```python
from build123d import *

# Parameters (mm, degrees)
BOSS_EXTRUDE2_DEPTH = 20
BOSS_EXTRUDE3_DEPTH = 2
BOSS_EXTRUDE4_START = 20
BOSS_EXTRUDE4_DEPTH = 2
CUT_EXTRUDE1_DEPTH  = 5
CUT_EXTRUDE2_DEPTH  = 5


with BuildPart() as part:
    # Sketch1 → Boss-Extrude2 (new body)
    with BuildSketch(Plane(origin=(0, 0, 0), x_dir=(0, 0, -1), z_dir=(1, 0, 0))):
        Polygon((0, 28), (0, 0), (28, 0), (28, 4), (4, 4), (4, 28), align=None)
    extrude(amount=BOSS_EXTRUDE2_DEPTH)

    # Sketch1_4 → Boss-Extrude3 (add)
    with BuildSketch(Plane(origin=(0, 0, 0), x_dir=(0, 0, -1), z_dir=(1, 0, 0))):
        Polygon((9.768810499, 28), (4, 28), (4, 4), (28, 4), (28, 9.768810499), (23.299944734, 9.768810499), (9.768810499, 23.299944734), align=None)
    extrude(amount=BOSS_EXTRUDE3_DEPTH)

    # Sketch1_5 → Boss-Extrude4 (add)
    with BuildSketch(Plane(origin=(0, 0, 0), x_dir=(0, 0, -1), z_dir=(1, 0, 0)).offset(BOSS_EXTRUDE4_START)):
        Polygon((9.768810499, 28), (4, 28), (4, 4), (28, 4), (28, 9.768810499), (23.299944734, 9.768810499), (9.768810499, 23.299944734), align=None)
    extrude(amount=-BOSS_EXTRUDE4_DEPTH)

    # Sketch2 → Cut-Extrude1 (cut, through all)
    with BuildSketch(Plane(origin=(0, 4, 0), x_dir=(1, 0, 0), z_dir=(0, 1, 0))):
        with BuildLine():
            Line((7.5, 12), (7.5, 20))
            ThreePointArc((7.5, 20), (10, 22.5), (12.5, 20))
            Line((12.5, 20), (12.5, 12))
            ThreePointArc((12.5, 12), (10, 9.5), (7.5, 12))
        make_face()
    extrude(amount=-CUT_EXTRUDE1_DEPTH, mode=Mode.SUBTRACT)

    # Sketch4 → Cut-Extrude2 (cut, through all)
    with BuildSketch(Plane(origin=(0, 0, -4), x_dir=(-1, 0, 0), z_dir=(0, 0, -1))):
        with BuildLine():
            Line((-12.5, 12), (-12.5, 20))
            ThreePointArc((-12.5, 20), (-10, 22.5), (-7.5, 20))
            Line((-7.5, 20), (-7.5, 12))
            ThreePointArc((-7.5, 12), (-10, 9.5), (-12.5, 12))
        make_face()
    extrude(amount=-CUT_EXTRUDE2_DEPTH, mode=Mode.SUBTRACT)


solid = part.part
```
Read the model definition and answer for the solid it produces. Units are mm, in the model's axes. A direction names the side the tool comes from. Give positions to 0.01 mm unless a question says otherwise; leave off trailing zeros. Write each loop counter-clockwise with the first axis right and the second up, starting at its lowest first coordinate (ties: lowest second). Pieces come first, ordered by that corner, then holes. Notation, with made-up numbers: (14.5, 39.25) -> (47.5, 39.25) arc R24 cw to (47.5, 62.25) -> close; hole circle Ø9 at (43, 46.25). An arc over 180 degrees is marked (long way). Answer as a JSON object with one key per item and string values.
1) Section A-A on x = 10 is taken. Write down the section's boundary in (y, z).
Findings below:
{"outline": "(0, -28) -> (4, -28) -> (4, -22.5) -> (0, -22.5) -> close; (0, -9.5) -> (4, -9.5) -> (4, -4) -> (9.5, -4) -> (9.5, 0) -> (0, 0) -> close; (22.5, -4) -> (28, -4) -> (28, 0) -> (22.5, 0) -> close"}
2) Section C-C on y = 5.75 is taken. Write down the section's boundary in (x, z), then the cut area to 3 significant figures.
Findings below:
{"outline": "(0, -28) -> (2, -28) -> (2, -4) -> (18, -4) -> (18, -28) -> (20, -28) -> (20, 0) -> (0, 0) -> close", "area": "176 mm^2"}
3) Section B-B on z = -17.5 is taken. Write down the section's boundary in (x, y), then the cut area to 3 significant figures.
Findings below:
{"outline": "(0, 0) -> (7.5, 0) -> (7.5, 4) -> (2, 4) -> (2, 15.57) -> (0, 15.57) -> close; (12.5, 0) -> (20, 0) -> (20, 15.57) -> (18, 15.57) -> (18, 4) -> (12.5, 4) -> close", "area": "106 mm^2"}
4) Section D-D on z = -4.5 is taken. Write down the section's boundary in (x, y), then the cut area to 3 significant figures.
Findings below:
{"outline": "(0, 0) -> (20, 0) -> (20, 28) -> (18, 28) -> (18, 4) -> (2, 4) -> (2, 28) -> (0, 28) -> close", "area": "176 mm^2"}
5) A tool of negligible diameter and unlimited length cuts with its end or side. For faces 4 (the cylindrical face through (10.1, 2, -9.5)), 5 (the cylindrical face through (9.9, 9.5, -2)), 6 (the flat face through (2, 14, -13)), 7 (the flat face through (19, 9.769, -26)), from which of +Z, -Z, +X, -X, +Y, -Y can it reach the whole face along a straight path? Write none if from no direction.
Findings below:
{"face 4": "+Y, -Y", "face 5": "+Z, -Z", "face 6": "-Z, +Y", "face 7": "-Z, +X, -X, +Y"}
6) Flat-ended cylindrical pins translate along their axes: pin 1 Ø5 at (x, y) = (10.5, 14.5) entering from -Z; pin 2 Ø4 at (x, z) = (12.5, -16.5) entering from +Y; pin 3 Ø2 at (x, z) = (19, -26.5) entering from +Y. Find the tip coordinate at first contact, or state that the pin passes through.
Findings below:
{"pin 1": "stops at z = -4", "pin 2": "stops at y = 4", "pin 3": "stops at y = 9.77"}
7) For a pull along X with two mould halves and no side action, classify faces 1 (the flat face through (12.5, 16, -2)), 2 (the flat face through (20, 11, -11)), 3 (the flat face through (7.6, 0, -10.7)) as pulls with the +X half, pulls with the -X half, needs draft (parallel to the pull), parting line crosses it, or undercut.
Findings below:
{"face 1": "undercut", "face 2": "pulls with the +X half", "face 3": "needs draft"}
8) Straight lines are drawn through the part: probe 1 along X at (y, z) = (8.25, -13.75); probe 2 along Z at (x, y) = (17, 25.75); probe 3 along Y at (x, z) = (13, -18.5). For each, find the intervals that lie inside material, in ascending order. Write a range as from..to.
Findings below:
{"probe 1": "x = 0..2, 18..20", "probe 2": "z = -4..0", "probe 3": "y = 0..4"}
